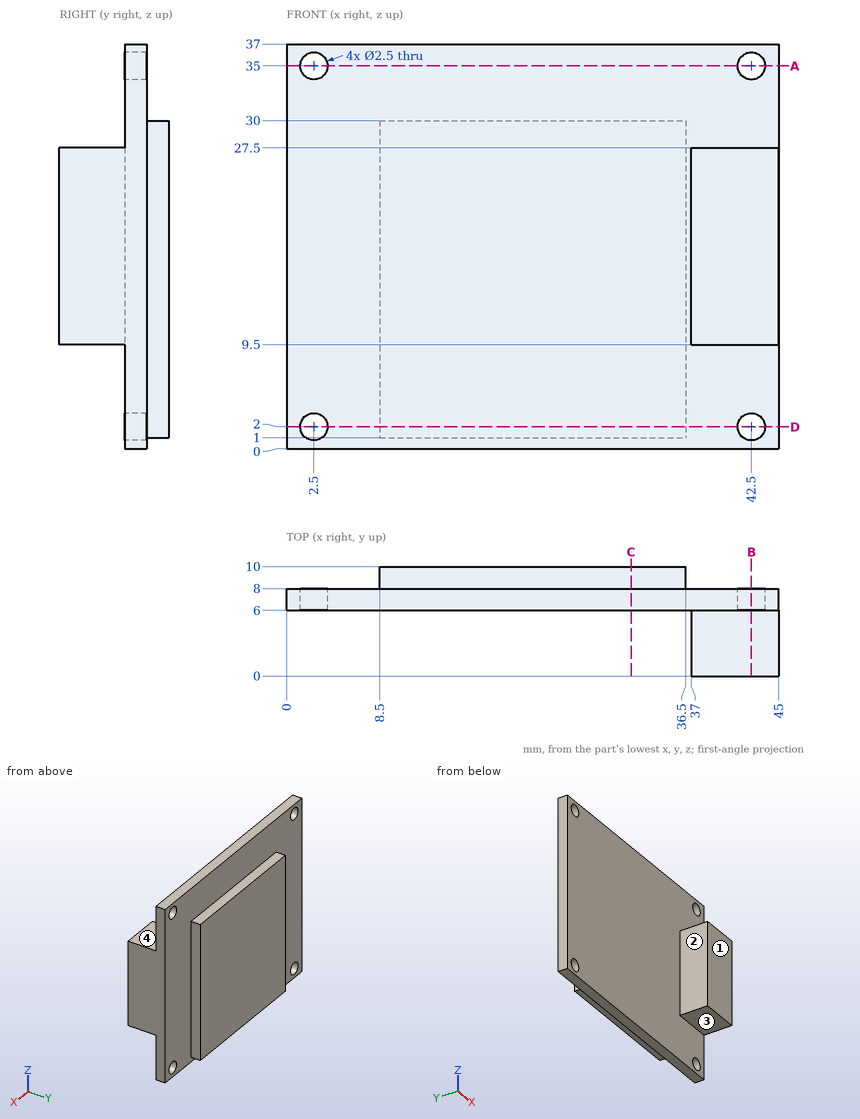
Input: dimensioned drawing with shaded views. Units: mm. Origin: part minimum x, y, z. A direction names the side the tool comes from. Round coordinates to 2 decimals unless told otherwise and drop trailing zeros. Loops run counter-clockwise (first coordinate to the right, second up) from the corner with the lowest first, then second, coordinate; pieces in that order, holes last. Notation, with made-up numbers: (-37.5, -21.5) -> (-20.5, -21.5) arc R16 ccw to (-20.5, -5.5) -> close; hole circle Ø4 at (-6.5, -25). An arc over 180 degrees is marked (long way). Use one line per item in the form item = value. Start each with the question number.
1) Section A-A on z = 35. Output: boundary loops of the cut face in (x, y), then the cut area to 3 significant figures.
2) First-contact query: P1, Ø3, axis at x = 42.5, z = 35, coming from the -Y side; P2, Ø1, axis at y = 9.5, z = 20, coming from the -X side; P3, Ø2, axis at x = 2.5, z = 35, coming from the +Y side; P4, Ø3, axis at x = 40.5, y = 3.5, coming from the +Z side. Flat tips, straight axial feed; report the tip coordinate or a pass-through.
3) Section B-B on x = 42.5. Output: boundary loops of the cut face in (y, z), then the cut area to 3 significant figures.
4) Line query: L1, parallel to X at y = 6.95, z = 35; L2, parallel to Y at x = 31.5, z = 28; L3, parallel to X at y = 9, z = 16.5. Output: solid intervals per line, ascending.
5) Section D-D on z = 2. Output: boundary loops of the cut face in (x, y).
6) Section C-C on x = 31.5. Output: boundary loops of the cut face in (y, z), then the cut area to 3 significant figures.
7) Access query for the marked faces 1, 2, 3 and 4. Directions: +Z, -Z, +X, -X, +Y, -Y. A direction counts if a zero-diameter tool reaches every point of the face in a straight line with its end or side. Return the directions, or none.
Response:
q1.outline = (0, 6) -> (1.25, 6) -> (1.25, 8) -> (0, 8) -> close; (3.75, 6) -> (41.25, 6) -> (41.25, 8) -> (3.75, 8) -> close; (43.75, 6) -> (45, 6) -> (45, 8) -> (43.75, 8) -> close
q1.area = 80.0 mm^2
q2.P1 = 6
q2.P2 = 8.5
q2.P3 = through
q2.P4 = 27.5
q3.outline = (0, 9.5) -> (6, 9.5) -> (6, 3.25) -> (8, 3.25) -> (8, 33.75) -> (6, 33.75) -> (6, 27.5) -> (0, 27.5) -> close; (6, 0) -> (8, 0) -> (8, 0.75) -> (6, 0.75) -> close; (6, 36.25) -> (8, 36.25) -> (8, 37) -> (6, 37) -> close
q3.area = 172 mm^2
q4.L1 = 0 to 1.25, 3.75 to 41.25, 43.75 to 45
q4.L2 = 6 to 10
q4.L3 = 8.5 to 36.5
q5.outline = (0, 6) -> (1.25, 6) -> (1.25, 8) -> (0, 8) -> close; (3.75, 6) -> (41.25, 6) -> (41.25, 8) -> (36.5, 8) -> (36.5, 10) -> (8.5, 10) -> (8.5, 8) -> (3.75, 8) -> close; (43.75, 6) -> (45, 6) -> (45, 8) -> (43.75, 8) -> close
q6.outline = (6, 0) -> (8, 0) -> (8, 1) -> (10, 1) -> (10, 30) -> (8, 30) -> (8, 37) -> (6, 37) -> close
q6.area = 132 mm^2
q7.face_1 = +Z, -Z, +X, -X, -Y
q7.face_2 = +Z, -Z, -X, -Y
q7.face_3 = -Z, +X, -X, -Y
q7.face_4 = +Z, +X, -X, -Y
